Could you check a few things on this model? Use its own coordinates, in mm. A direction names the side the tool comes from. Coordinates: 2 decimals unless noted, no trailing zeros. Loops run counter-clockwise (first coordinate to the right, second up) from the corner with the lowest first, then second, coordinate; pieces in that order, holes last.
1) Imagine slicing it at D-D on y = 1. Please give me the cut outline in (x, z).
2) Thinking about a two-plate mould opening in Z: for faces 1 (the face through (-3.1, 3.9, -39.2)), 2 (the face through (-24, 4, -44)), 3 (the face through (-40.393, 3.789, -5.07)), which applies, released by +Z, released by -Z, zero draft, split by the parting line, or undercut?
3) If I drill on line 1 along X through (y, z) = (4, -40.5); line 2 along Z through (x, y) = (-4, 6.25); line 3 along Y through (x, z) = (-42, -7), over which ranges is the centre line in solid material (lowest first)?
4) Imagine slicing it at A-A on z = -38. Please give me the cut outline in (x, y).
5) Imagine slicing it at C-C on z = -22. Please give me the cut outline in (x, y).
6) For faces 4 (the face through (-42, 4, -34)), 5 (the face through (-45.972, 3.513, -20.454)), 6 (the face through (-10.63, 4.87, -5.07)), which set-ups out of +Z, -Z, +X, -X, +Y, -Y let a thin tool reach every point of the face, with its end or its side?
7) Imagine slicing it at B-B on x = -4. Please give me the cut outline in (y, z).
8) Will these pins go through, and if not, where does the flat tip stop? P1, Ø3, axis at y = 4, z = -22, coming from the +X side; P2, Ø3, axis at x = -20.41, z = -13, coming from the -Y side; P3, Ø2.5, axis at x = -12, y = 4, coming from the -Z side; P4, Ø3, axis at x = -42, y = 4, coming from the +Z side.
Autodesk Inventor part; units mm, degrees
ref_plane "Arbeitsebene1" through (0, 0, -22) normal (0, 0, 1) x (1, 0, 0)
ref_plane "YZ Plane" through (0, 0, 0) normal (1, 0, 0) x (0, 1, 0)
ref_plane "XZ Plane" through (0, 0, 0) normal (0, 1, 0) x (-1, 0, 0)
sketch "Skizze1" plane through (0, 0, 0) normal (0, 1, 0) x (-1, 0, 0)
  line L0 (0, 0) -> (48, 0)
  line L1 (48, 0) -> (48, -44)
  line L2 (48, -44) -> (0, -44)
  line L3 (0, -44) -> (0, 0)
  dimension "d0" = 44
  dimension "d1" = 48
extrude "Extrusion1" add sketch "Skizze1" along normal blind 8
sketch "Skizze2" plane through (0, 8, 0) normal (0, 1, 0) x (1, 0, 0)
  circle A0 centre (-36, 22) radius 5
  circle A1 centre (-20.4115, 13) radius 2
  circle A2 centre (-20.4115, 31) radius 3
  line L0 (0, 0) -> (0, 44)
  line L1 (0, 22) -> (-47.9314, 22) construction
  line L2 (-48, 44) -> (-48, 0)
  dimension "d4" = 9
  dimension "d5" = 12
  dimension "d6" = 10
  dimension "d7" = 18
  dimension "d8" = 4
  dimension "d9" = 6
extrude "Extrusion2" cut sketch "Skizze2" against normal up to surface (8 mm away)
sketch "Skizze3" plane through (-48, 0, -44) normal (-1, 0, 0) x (0, 0, 1)
  line L0 (44, 0) -> (44, 8)
  line L1 (0, 0) -> (44, 0)
  point P0 (22, 4)
  point P1 (44, 4)
  point P2 (22, 0)
hole "Bohrung1" at (-48, 4, -22) direction (1, 0, 0) diameter 3.242 depth 4
sketch "Skizze4" plane through (0, 8, 0) normal (0, 1, 0) x (1, 0, 0)
  line L0 (0, 0) -> (0, 44)
  line L1 (-48, 0) -> (0, 0)
  point P0 (-4, 6)
  point P1 (-4, 38)
  dimension "d26" = 4
  dimension "d27" = 6
  dimension "d28" = 32
hole "Bohrung2" at (-4, 8, -6) at (-4, 8, -38) direction (0, -1, 0) diameter 3 depth 8
sketch "Skizze5" plane through (0, 0, -44) normal (0, 0, -1) x (-1, 0, 0)
  line L0 (48, 0) -> (48, 8)
  line L1 (0, 0) -> (0, 8)
  point P0 (12, 4)
  point P1 (42, 4)
  point P2 (48, 4)
  dimension "d36" = 30
  dimension "d37" = 12
hole "Bohrung3" at (-12, 4, -44) at (-42, 4, -44) direction (0, 0, 1) diameter 3.242 depth 10
ref_plane "Arbeitsebene1" through (0, 0, -22) normal (0, 0, 1) x (1, 0, 0)
mirror "Spiegeln1" about plane through (0, 0, -22) normal (0, 0, 1) of "Bohrung3"
properties part number "1014"
Filled in:
1. outline: (-48, -44) - (0, -44) - (0, 0) - (-48, 0) - close; hole circle Ø10 at (-36, -22); hole circle Ø6 at (-20.41, -31); hole circle Ø4 at (-20.41, -13); hole circle Ø3 at (-4, -38); hole circle Ø3 at (-4, -6)
2. face 1: undercut
2. face 2: released by -Z
2. face 3: zero draft
3. line 1: x = -48 to -43.62, -40.38 to -13.62, -10.38 to 0
3. line 2: z = -44 to -39.5, -36.5 to -7.5, -4.5 to 0
3. line 3: y = 0 to 2.38, 5.62 to 8
4. outline: (-48, 0) - (-5.5, 0) - (-5.5, 8) - (-48, 8) - close; (-2.5, 0) - (0, 0) - (0, 8) - (-2.5, 8) - close; hole circle Ø3.24 at (-42, 4); hole circle Ø3.24 at (-12, 4)
5. outline: (-48, 0) - (-41, 0) - (-41, 8) - (-48, 8) - (-48, 5.62) - (-44, 5.62) - (-44, 2.38) - (-48, 2.38) - close; (-31, 0) - (0, 0) - (0, 8) - (-31, 8) - close
6. face 4: -Z
6. face 5: -X
6. face 6: +Z
7. outline: (0, -44) - (8, -44) - (8, -39.5) - (0, -39.5) - close; (0, -36.5) - (8, -36.5) - (8, -7.5) - (0, -7.5) - close; (0, -4.5) - (8, -4.5) - (8, 0) - (0, 0) - close
8. P1: stops at x = 0
8. P2: passes through
8. P3: stops at z = -34
8. P4: stops at z = -10
